Verification items for the finished model (mm, model axes). Give positions to 0.01 mm unless a question says otherwise; leave off trailing zeros. Order: outer loops, then holes, each group sorted by start corner. A loop starts at its lowest first (then second) coordinate and runs counter-clockwise, first axis right, second up. Notation, with made-up numbers: M 67.25,34 L 109.25,34 A20 ccw 109.25,69 Z; hole C 57,89.25 d5. An arc over 180 degrees is marked long. Answer as a JSON object with one key per item and string values.
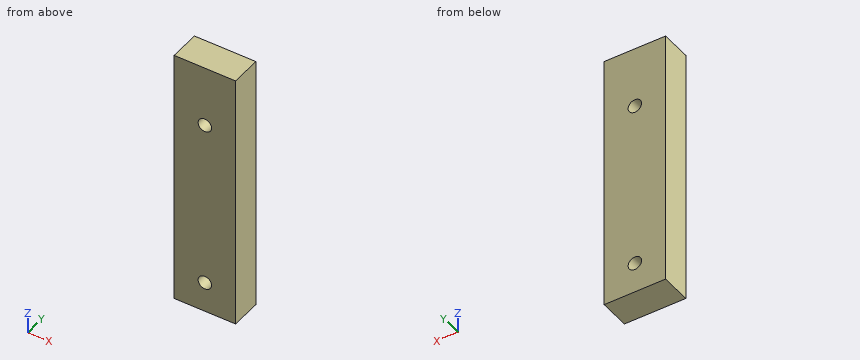
```python
from build123d import *

# Parameters (mm, degrees)
SKETCH1_W           = 304.8
SKETCH1_H           = 304.8
BOSS_EXTRUDE1_DEPTH = 6.35
CUT_EXTRUDE2_DEPTH  = 6.35
SKETCH3_R           = 1.3890625
CUT_EXTRUDE3_DEPTH  = 306.130549929


with BuildPart() as part:
    # Sketch1 → Boss-Extrude1 (new body)
    with BuildSketch(Plane(origin=(0, 0, 0), x_dir=(1, 0, 0), z_dir=(0, 1, 0))):
        with Locations((152.4, 152.4)):
            Rectangle(SKETCH1_W, SKETCH1_H)
    extrude(amount=BOSS_EXTRUDE1_DEPTH)

    # Sketch2 → Cut-Extrude2 (cut)
    with BuildSketch(Plane(origin=(0, 6.35, 0), x_dir=(1, 0, 0), z_dir=(0, 1, 0))):
        Polygon((12.7, 304.8), (12.7, 250.825), (0, 250.825), (0, 0), (304.8, 0), (304.8, 304.8), align=None)
    extrude(amount=-CUT_EXTRUDE2_DEPTH, mode=Mode.SUBTRACT)

    # Sketch3 → Cut-Extrude3 (cut, through all)
    with BuildSketch(Plane(origin=(0, 6.35, 0), x_dir=(1, 0, 0), z_dir=(0, 1, 0))):
        with Locations(Location((6.35, 263.525, 0), (0, 0, 270))):
            Circle(SKETCH3_R)
        with Locations(Location((6.35, 298.45, 0), (0, 0, 270))):
            Circle(SKETCH3_R)
    extrude(amount=-CUT_EXTRUDE3_DEPTH, mode=Mode.SUBTRACT)


solid = part.part
```
Q1. Section check C-C on y = 2. Record the cut outline in (x, z) (3 decimals), then the cut area to 3 significant figures.
Resolved:
{"outline": "M 0,-304.8 L 12.7,-304.8 L 12.7,-250.825 L 0,-250.825 Z; hole C 6.35,-298.45 d2.778; hole C 6.35,-263.525 d2.778", "area": "673 mm²"}
Q2. Section check B-B on x = 6.35. Record the cut outline in (y, z) (3 decimals).
Resolved:
{"outline": "M 0,-304.8 L 6.35,-304.8 L 6.35,-299.839 L 0,-299.839 Z; M 0,-297.061 L 6.35,-297.061 L 6.35,-264.914 L 0,-264.914 Z; M 0,-262.136 L 6.35,-262.136 L 6.35,-250.825 L 0,-250.825 Z"}
Q3. Section check A-A on z = -298.45. Record the cut outline in (x, y).
Resolved:
{"outline": "M 0,0 L 4.96,0 L 4.96,6.35 L 0,6.35 Z; M 7.74,0 L 12.7,0 L 12.7,6.35 L 7.74,6.35 Z"}
Q4. Material ranges on L1, parallel to Z at x = 6.5, y = 2.5 (3 decimals); L2, parallel to X at y = 3, z = -298.45, recorded low to high.
Resolved:
{"L1": "z = -304.8 to -299.831, -297.069 to -264.906, -262.144 to -250.825", "L2": "x = 0 to 4.96, 7.74 to 12.7"}
